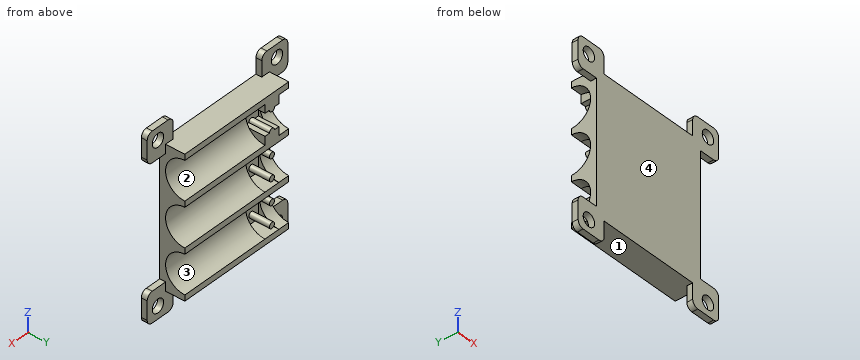
```python
from build123d import *

# Parameters (mm, degrees)
BOSS_EXTRUDE1_DEPTH = 41
BOSS_EXTRUDE2_REACH = 50.098
SKETCH2_R           = 1
SKETCH4_W           = 5.5
SKETCH4_H           = 13.1
SKETCH4_R           = 1
CUT_EXTRUDE1_DEPTH  = 7
SKETCH5_R           = 2.25
BOSS_EXTRUDE3_DEPTH = 2
BOSS_EXTRUDE4_REACH = 59.938
SKETCH6_W           = 5.5
SKETCH6_H           = 2.85
CUT_EXTRUDE2_DEPTH  = 7


with BuildPart() as part:
    # Sketch1 → Boss-Extrude1 (new body)
    with BuildSketch(Plane(origin=(0, 0, 0), x_dir=(0, 0, -1), z_dir=(1, 0, 0))):
        with BuildLine():
            Line((-8.55, 0), (-6.55, 0))
            ThreePointArc((-6.55, 0), (0, -6.55), (6.55, 0))
            Line((6.55, 0), (8.55, 0))
            ThreePointArc((8.55, 0), (15.1, -6.55), (21.65, 0))
            Line((21.65, 0), (23.65, 0))
            Line((23.65, 0), (23.65, -8.55))
            Line((23.65, -8.55), (-23.65, -8.55))
            Line((-23.65, -8.55), (-23.65, 0))
            Line((-23.65, 0), (-21.65, 0))
            ThreePointArc((-21.65, 0), (-15.1, -6.55), (-8.55, 0))
        make_face()
    extrude(amount=BOSS_EXTRUDE1_DEPTH)

    # Sketch2 → Boss-Extrude2 (add, up to next)
    with BuildSketch(Plane(origin=(0, 0, 0), x_dir=(1, 0, 0), z_dir=(0, 1, 0)), mode=Mode.PRIVATE) as boss_extrude2_sk1:
        with Locations(Location((6.6, 3.7, 0), (0, 0, 270))):
            Circle(SKETCH2_R)
    boss_extrude2_tool1 = extrude(boss_extrude2_sk1.sketch, amount=-BOSS_EXTRUDE2_REACH, mode=Mode.PRIVATE) - part.part
    # Sketch2 → Boss-Extrude2 (add, up to next)
    with BuildSketch(Plane(origin=(0, 0, 0), x_dir=(1, 0, 0), z_dir=(0, 1, 0)), mode=Mode.PRIVATE) as boss_extrude2_sk2:
        with Locations(Location((6.6, -3.7, 0), (0, 0, 270))):
            Circle(SKETCH2_R)
    boss_extrude2_tool2 = extrude(boss_extrude2_sk2.sketch, amount=-BOSS_EXTRUDE2_REACH, mode=Mode.PRIVATE) - part.part
    # Sketch2 → Boss-Extrude2 (add, up to next)
    with BuildSketch(Plane(origin=(0, 0, 0), x_dir=(1, 0, 0), z_dir=(0, 1, 0)), mode=Mode.PRIVATE) as boss_extrude2_sk3:
        with Locations(Location((6.6, -11.4, 0), (0, 0, 270))):
            Circle(SKETCH2_R)
    boss_extrude2_tool3 = extrude(boss_extrude2_sk3.sketch, amount=-BOSS_EXTRUDE2_REACH, mode=Mode.PRIVATE) - part.part
    # Sketch2 → Boss-Extrude2 (add, up to next)
    with BuildSketch(Plane(origin=(0, 0, 0), x_dir=(1, 0, 0), z_dir=(0, 1, 0)), mode=Mode.PRIVATE) as boss_extrude2_sk4:
        with Locations(Location((6.6, -18.8, 0), (0, 0, 270))):
            Circle(SKETCH2_R)
    boss_extrude2_tool4 = extrude(boss_extrude2_sk4.sketch, amount=-BOSS_EXTRUDE2_REACH, mode=Mode.PRIVATE) - part.part
    # Sketch2 → Boss-Extrude2 (add, up to next)
    with BuildSketch(Plane(origin=(0, 0, 0), x_dir=(1, 0, 0), z_dir=(0, 1, 0)), mode=Mode.PRIVATE) as boss_extrude2_sk5:
        with Locations(Location((6.6, 18.8, 0), (0, 0, 270))):
            Circle(SKETCH2_R)
    boss_extrude2_tool5 = extrude(boss_extrude2_sk5.sketch, amount=-BOSS_EXTRUDE2_REACH, mode=Mode.PRIVATE) - part.part
    # Sketch2 → Boss-Extrude2 (add, up to next)
    with BuildSketch(Plane(origin=(0, 0, 0), x_dir=(1, 0, 0), z_dir=(0, 1, 0)), mode=Mode.PRIVATE) as boss_extrude2_sk6:
        with Locations(Location((6.6, 11.4, 0), (0, 0, 270))):
            Circle(SKETCH2_R)
    boss_extrude2_tool6 = extrude(boss_extrude2_sk6.sketch, amount=-BOSS_EXTRUDE2_REACH, mode=Mode.PRIVATE) - part.part
    add(boss_extrude2_tool1.solids().sort_by_distance((6.6, 0, -3.7))[0])
    add(boss_extrude2_tool2.solids().sort_by_distance((6.6, 0, 3.7))[0])
    add(boss_extrude2_tool3.solids().sort_by_distance((6.6, 0, 11.4))[0])
    add(boss_extrude2_tool4.solids().sort_by_distance((6.6, 0, 18.8))[0])
    add(boss_extrude2_tool5.solids().sort_by_distance((6.6, 0, -18.8))[0])
    add(boss_extrude2_tool6.solids().sort_by_distance((6.6, 0, -11.4))[0])

    # Sketch4 → Cut-Extrude1 (cut)
    # profile 1 of 3: a face of its own
    with BuildSketch(Plane(origin=(0, 0, 0), x_dir=(1, 0, 0), z_dir=(0, 1, 0))):
        with Locations((6.6, 0)):
            Rectangle(SKETCH4_W, SKETCH4_H)
        with Locations(Location((6.6, 3.7, 0), (0, 0, 270))):
            Circle(SKETCH4_R, mode=Mode.SUBTRACT)
        with Locations(Location((6.6, -3.7, 0), (0, 0, 270))):
            Circle(SKETCH4_R, mode=Mode.SUBTRACT)
    # profile 2 of 3: a face of its own
    with BuildSketch(Plane(origin=(0, 0, 0), x_dir=(1, 0, 0), z_dir=(0, 1, 0))):
        with Locations((6.6, -15.1)):
            Rectangle(SKETCH4_W, SKETCH4_H)
        with Locations(Location((6.6, -11.4, 0), (0, 0, 90))):
            Circle(SKETCH4_R, mode=Mode.SUBTRACT)
        with Locations(Location((6.6, -18.8, 0), (0, 0, 90))):
            Circle(SKETCH4_R, mode=Mode.SUBTRACT)
    # profile 3 of 3: a face of its own
    with BuildSketch(Plane(origin=(0, 0, 0), x_dir=(1, 0, 0), z_dir=(0, 1, 0))):
        with Locations((6.6, 15.1)):
            Rectangle(SKETCH4_W, SKETCH4_H)
        with Locations(Location((6.6, 11.4, 0), (0, 0, 90))):
            Circle(SKETCH4_R, mode=Mode.SUBTRACT)
        with Locations(Location((6.6, 18.8, 0), (0, 0, 90))):
            Circle(SKETCH4_R, mode=Mode.SUBTRACT)
    extrude(amount=-CUT_EXTRUDE1_DEPTH, mode=Mode.SUBTRACT)

    # Sketch5 → Boss-Extrude3 (add)
    # profile 1 of 4: a face of its own
    with BuildSketch(Plane.XZ.offset(8.55)):
        with BuildLine():
            Line((0, 23.65), (0, 20.65))
            Line((0, 20.65), (-5.25520382, 20.65))
            ThreePointArc((-5.25520382, 20.65), (-6.669417382, 21.235786438), (-7.25520382, 22.65))
            Line((-7.25520382, 22.65), (-7.25520382, 28.90520382))
            ThreePointArc((-7.25520382, 28.90520382), (-6.669417382, 30.319417382), (-5.25520382, 30.90520382))
            Line((-5.25520382, 30.90520382), (1, 30.90520382))
            ThreePointArc((1, 30.90520382), (2.414213562, 30.319417382), (3, 28.90520382))
            Line((3, 28.90520382), (3, 23.65))
            Line((3, 23.65), (0, 23.65))
        make_face()
        with Locations(Location((-3.00520382, 26.65520382, 0), (0, 0, 270))):
            Circle(SKETCH5_R, mode=Mode.SUBTRACT)
    # profile 2 of 4: a face of its own
    with BuildSketch(Plane.XZ.offset(8.55)):
        with BuildLine():
            Line((0, -23.65), (3, -23.65))
            Line((3, -23.65), (3, -28.90520382))
            ThreePointArc((3, -28.90520382), (2.414213562, -30.319417382), (1, -30.90520382))
            Line((1, -30.90520382), (-5.25520382, -30.90520382))
            ThreePointArc((-5.25520382, -30.90520382), (-6.669417382, -30.319417382), (-7.25520382, -28.90520382))
            Line((-7.25520382, -28.90520382), (-7.25520382, -22.65))
            ThreePointArc((-7.25520382, -22.65), (-6.669417382, -21.235786438), (-5.25520382, -20.65))
            Line((-5.25520382, -20.65), (0, -20.65))
            Line((0, -20.65), (0, -23.65))
        make_face()
        with Locations(Location((-3.00520382, -26.65520382, 0), (0, 0, 90))):
            Circle(SKETCH5_R, mode=Mode.SUBTRACT)
    # profile 3 of 4: a face of its own
    with BuildSketch(Plane.XZ.offset(8.55)):
        with BuildLine():
            Line((41, -23.65), (41, -20.65))
            Line((41, -20.65), (46.25520382, -20.65))
            ThreePointArc((46.25520382, -20.65), (47.669417382, -21.235786438), (48.25520382, -22.65))
            Line((48.25520382, -22.65), (48.25520382, -28.90520382))
            ThreePointArc((48.25520382, -28.90520382), (47.669417382, -30.319417382), (46.25520382, -30.90520382))
            Line((46.25520382, -30.90520382), (40, -30.90520382))
            ThreePointArc((40, -30.90520382), (38.585786438, -30.319417382), (38, -28.90520382))
            Line((38, -28.90520382), (38, -23.65))
            Line((38, -23.65), (41, -23.65))
        make_face()
        with Locations(Location((44.00520382, -26.65520382, 0), (0, 0, 270))):
            Circle(SKETCH5_R, mode=Mode.SUBTRACT)
    # profile 4 of 4: a face of its own
    with BuildSketch(Plane.XZ.offset(8.55)):
        with BuildLine():
            Line((41, 23.65), (38, 23.65))
            Line((38, 23.65), (38, 28.90520382))
            ThreePointArc((38, 28.90520382), (38.585786438, 30.319417382), (40, 30.90520382))
            Line((40, 30.90520382), (46.25520382, 30.90520382))
            ThreePointArc((46.25520382, 30.90520382), (47.669417382, 30.319417382), (48.25520382, 28.90520382))
            Line((48.25520382, 28.90520382), (48.25520382, 22.65))
            ThreePointArc((48.25520382, 22.65), (47.669417382, 21.235786438), (46.25520382, 20.65))
            Line((46.25520382, 20.65), (41, 20.65))
            Line((41, 20.65), (41, 23.65))
        make_face()
        with Locations(Location((44.00520382, 26.65520382, 0), (0, 0, 90))):
            Circle(SKETCH5_R, mode=Mode.SUBTRACT)
    extrude(amount=-BOSS_EXTRUDE3_DEPTH)

    # Boss-Extrude4: up to this face of the body (flat: up to its plane)
    boss_extrude4_end = Plane(part.part.faces().sort_by_distance((6.6, -7, -15.1))[0])
    # Sketch6 → Boss-Extrude4 (add, up to the picked face)
    with BuildSketch(Plane(origin=(0, 0, 0), x_dir=(1, 0, 0), z_dir=(0, 1, 0)), mode=Mode.PRIVATE) as boss_extrude4_sk1:
        with Locations((6.6, -5.125)):
            Rectangle(SKETCH6_W, SKETCH6_H)
    boss_extrude4_tool1 = split(extrude(boss_extrude4_sk1.sketch, amount=-BOSS_EXTRUDE4_REACH, mode=Mode.PRIVATE), bisect_by=boss_extrude4_end, keep=Keep.BOTH, mode=Mode.PRIVATE)
    # Sketch6 → Boss-Extrude4 (add, up to the picked face)
    with BuildSketch(Plane(origin=(0, 0, 0), x_dir=(1, 0, 0), z_dir=(0, 1, 0)), mode=Mode.PRIVATE) as boss_extrude4_sk2:
        with Locations((6.6, 5.125)):
            Rectangle(SKETCH6_W, SKETCH6_H)
    boss_extrude4_tool2 = split(extrude(boss_extrude4_sk2.sketch, amount=-BOSS_EXTRUDE4_REACH, mode=Mode.PRIVATE), bisect_by=boss_extrude4_end, keep=Keep.BOTH, mode=Mode.PRIVATE)
    # Sketch6 → Boss-Extrude4 (add, up to the picked face)
    with BuildSketch(Plane(origin=(0, 0, 0), x_dir=(1, 0, 0), z_dir=(0, 1, 0)), mode=Mode.PRIVATE) as boss_extrude4_sk3:
        with Locations((6.6, -20.225)):
            Rectangle(SKETCH6_W, SKETCH6_H)
    boss_extrude4_tool3 = split(extrude(boss_extrude4_sk3.sketch, amount=-BOSS_EXTRUDE4_REACH, mode=Mode.PRIVATE), bisect_by=boss_extrude4_end, keep=Keep.BOTH, mode=Mode.PRIVATE)
    # Sketch6 → Boss-Extrude4 (add, up to the picked face)
    with BuildSketch(Plane(origin=(0, 0, 0), x_dir=(1, 0, 0), z_dir=(0, 1, 0)), mode=Mode.PRIVATE) as boss_extrude4_sk4:
        with Locations((6.6, -9.975)):
            Rectangle(SKETCH6_W, SKETCH6_H)
    boss_extrude4_tool4 = split(extrude(boss_extrude4_sk4.sketch, amount=-BOSS_EXTRUDE4_REACH, mode=Mode.PRIVATE), bisect_by=boss_extrude4_end, keep=Keep.BOTH, mode=Mode.PRIVATE)
    # Sketch6 → Boss-Extrude4 (add, up to the picked face)
    with BuildSketch(Plane(origin=(0, 0, 0), x_dir=(1, 0, 0), z_dir=(0, 1, 0)), mode=Mode.PRIVATE) as boss_extrude4_sk5:
        with Locations((6.6, 9.975)):
            Rectangle(SKETCH6_W, SKETCH6_H)
    boss_extrude4_tool5 = split(extrude(boss_extrude4_sk5.sketch, amount=-BOSS_EXTRUDE4_REACH, mode=Mode.PRIVATE), bisect_by=boss_extrude4_end, keep=Keep.BOTH, mode=Mode.PRIVATE)
    # Sketch6 → Boss-Extrude4 (add, up to the picked face)
    with BuildSketch(Plane(origin=(0, 0, 0), x_dir=(1, 0, 0), z_dir=(0, 1, 0)), mode=Mode.PRIVATE) as boss_extrude4_sk6:
        with Locations((6.6, 20.225)):
            Rectangle(SKETCH6_W, SKETCH6_H)
    boss_extrude4_tool6 = split(extrude(boss_extrude4_sk6.sketch, amount=-BOSS_EXTRUDE4_REACH, mode=Mode.PRIVATE), bisect_by=boss_extrude4_end, keep=Keep.BOTH, mode=Mode.PRIVATE)
    add(boss_extrude4_tool1.solids().sort_by(Axis((6.6, 0, 5.125), (0, -1, 0)))[0])
    add(boss_extrude4_tool2.solids().sort_by(Axis((6.6, 0, -5.125), (0, -1, 0)))[0])
    add(boss_extrude4_tool3.solids().sort_by(Axis((6.6, 0, 20.225), (0, -1, 0)))[0])
    add(boss_extrude4_tool4.solids().sort_by(Axis((6.6, 0, 9.975), (0, -1, 0)))[0])
    add(boss_extrude4_tool5.solids().sort_by(Axis((6.6, 0, -9.975), (0, -1, 0)))[0])
    add(boss_extrude4_tool6.solids().sort_by(Axis((6.6, 0, -20.225), (0, -1, 0)))[0])

    # Sketch7 → Cut-Extrude2 (cut)
    with BuildSketch(Plane(origin=(0, 0, 0), x_dir=(1, 0, 0), z_dir=(0, 1, 0))):
        with BuildLine():
            Line((5.6, 3.7), (3.85, 3.7))
            Line((3.85, 3.7), (3.85, 6.55))
            Line((3.85, 6.55), (9.35, 6.55))
            Line((9.35, 6.55), (9.35, 3.7))
            Line((9.35, 3.7), (7.6, 3.7))
            ThreePointArc((7.6, 3.7), (6.6, 4.7), (5.6, 3.7))
        make_face()
        with BuildLine():
            Line((7.6, -3.7), (9.35, -3.7))
            Line((9.35, -3.7), (9.35, -6.55))
            Line((9.35, -6.55), (3.85, -6.55))
            Line((3.85, -6.55), (3.85, -3.7))
            Line((3.85, -3.7), (5.6, -3.7))
            ThreePointArc((5.6, -3.7), (6.6, -4.7), (7.6, -3.7))
        make_face()
        with BuildLine():
            Line((5.6, 18.8), (3.85, 18.8))
            Line((3.85, 18.8), (3.85, 21.65))
            Line((3.85, 21.65), (9.35, 21.65))
            Line((9.35, 21.65), (9.35, 18.8))
            Line((9.35, 18.8), (7.6, 18.8))
            ThreePointArc((7.6, 18.8), (6.6, 19.8), (5.6, 18.8))
        make_face()
        with BuildLine():
            Line((7.6, 11.4), (9.35, 11.4))
            Line((9.35, 11.4), (9.35, 8.55))
            Line((9.35, 8.55), (3.85, 8.55))
            Line((3.85, 8.55), (3.85, 11.4))
            Line((3.85, 11.4), (5.6, 11.4))
            ThreePointArc((5.6, 11.4), (6.6, 10.4), (7.6, 11.4))
        make_face()
    extrude(amount=-CUT_EXTRUDE2_DEPTH, mode=Mode.SUBTRACT)


solid = part.part
```
The listing builds one solid part. Answer for the finished solid, in the listing's coordinates (mm). Face numbers are marked on the shaded views. A direction names the side the tool comes from. Give positions to 0.01 mm unless a question says otherwise; leave off trailing zeros. Write each loop counter-clockwise with the first axis right and the second up, starting at its lowest first coordinate (ties: lowest second). Pieces come first, ordered by that corner, then holes. Notation, with made-up numbers: (29.25, -6.75) - (64.25, -6.75) arc R26 cw to (64.25, 11.25) - close; hole circle Ø2 at (-15.75, -33.5). An arc over 180 degrees is marked (long way). Use one line per item in the form item = value. Start each with the question number.
1) Consider line 1 along X through (y, z) = (-2.5, 6.5); line 2 along Z through (x, y) = (36, -2.75); line 3 along Z through (x, y) = (30, -5.5). Determine where each line is inside the solid, lowest interval first. Write a range as from..to.
2) Flat-ended cylindrical pins translate along their axes: pin 1 Ø3 at (x, z) = (-2, 28) entering from +Y; pin 2 Ø1.3 at (y, z) = (-6.5, 15) entering from +X; pin 3 Ø2.5 at (y, z) = (-5.5, 3) entering from -X; pin 4 Ø3 at (y, z) = (-3, -15) entering from +X. Find the tip coordinate at first contact, or state that the pin passes through.
3) The mould has two halves that part along X. Classify the marked faces 1 and 2: pulls with the +X half, pulls with the -X half, needs draft (parallel to the pull), parting line crosses it, or undercut.
4) A tool of negligible diameter and unlimited length cuts with its end or side. For the marked faces 3 and 4, from which of +Z, -Z, +X, -X, +Y, -Y can it reach the whole face along a straight path? Write none if from no direction.
5) Find section A-A on z = -27. Determine the outline of the cut face in (x, y).
6) Find section C-C on z = 3.7. Determine the outline of the cut face in (x, y).
7) Find section D-D on y = -2.75. Count the separate pieces of the cut face and the enclosed holes in it, plus the area to 3 significant figures.
Geometry results:
q1.line_1 = 0..3.85, 9.35..41
q1.line_2 = -23.65..-21.04, -9.16..-5.94, 5.94..9.16, 21.04..23.65
q1.line_3 = -23.65..-18.66, -11.54..-3.56, 3.56..11.54, 18.66..23.65
q2.pin_1 = -6.55
q2.pin_2 = 41
q2.pin_3 = 0
q2.pin_4 = through
q3.face_1 = undercut
q3.face_2 = needs draft
q4.face_3 = +X, +Y
q4.face_4 = +Z, -Z, +X, -X, -Y
q5.outline = (-7.26, -8.55) - (-5.23, -8.55) - (-5.23, -6.55) - (-7.26, -6.55) - close; (-0.78, -8.55) - (3, -8.55) - (3, -6.55) - (-0.78, -6.55) - close; (38, -8.55) - (41.78, -8.55) - (41.78, -6.55) - (38, -6.55) - close; (46.23, -8.55) - (48.26, -8.55) - (48.26, -6.55) - (46.23, -6.55) - close
q6.outline = (0, -8.55) - (41, -8.55) - (41, -5.4) - (9.35, -5.4) - (9.35, -7) - (7.6, -7) - (7.6, 0) - (5.6, 0) - (5.6, -7) - (3.85, -7) - (3.85, -5.4) - (0, -5.4) - close
q7.separate_pieces = 8
q7.enclosed_holes = 0
q7.area = 504 mm2
